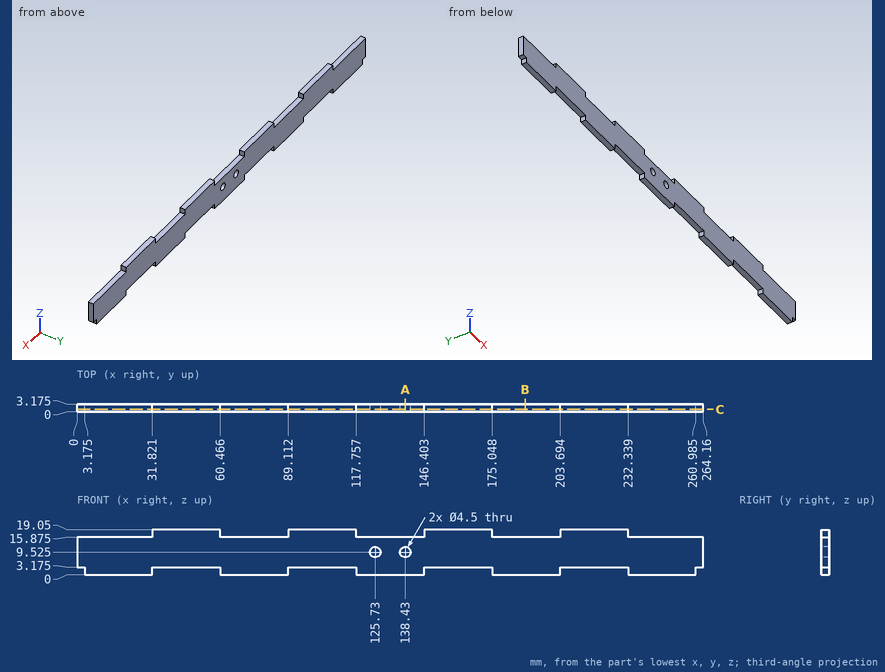
Input: dimensioned drawing with shaded views. Units: mm. Origin: part minimum x, y, z. Give positions to 0.01 mm unless a question says otherwise; leave off trailing zeros. Order: outer loops, then holes, each group sorted by start corner. A loop starts at its lowest first (then second) coordinate and runs counter-clockwise, first axis right, second up.
(1) Section query A-A (x = 138.43). Return the cut outline in (y, z) (1 decimal), plus the area to 3 significant figures.
(2) Contact query for flat-ended pins moving along their axis: P1, Ø1, axis at y = 2, z = 18, coming from the +X side; P2, Ø1.6, axis at y = 1.5, z = 17, coming from the -X side; P3, Ø1.6, axis at x = 213, y = 2.5, coming from the -Z side (3 decimals). Output: stop coordinate, or through.
(3) Material intervals for line 1 along X through (y, z) = (1.15, 2.75) (1 decimal); line 2 along X through (y, z) = (3, 9.25); line 3 along X through (y, z) = (1.8, 16.5), sorted ascending.
(4) Section query B-B (x = 189). Return the cut outline in (y, z) (1 decimal), plus the area to 3 significant figures.
(5) Section query C-C (y = 0.95). State how many separate pieces and enclosed holes the cut face has, plus the area to 3 significant figures.
Outcome:
1. outline: (0, 0) - (3.2, 0) - (3.2, 7.3) - (0, 7.3) - close; (0, 11.8) - (3.2, 11.8) - (3.2, 15.9) - (0, 15.9) - close
1. area: 36.1 mm2
2. P1: stops at x = 232.34
2. P2: stops at x = 31.82
2. P3: stops at z = 3.175
3. line 1: x = 3.2 to 31.8, 60.5 to 89.1, 117.8 to 146.4, 175 to 203.7, 232.3 to 261
3. line 2: x = 0 to 123.5, 127.96 to 136.2, 140.66 to 264.16
3. line 3: x = 31.82 to 60.47, 89.11 to 117.76, 146.4 to 175.05, 203.69 to 232.34
4. outline: (0, 0) - (3.2, 0) - (3.2, 15.9) - (0, 15.9) - close
4. area: 50.4 mm2
5. separate pieces: 1
5. enclosed holes: 2
5. area: 4,140 mm2
